```python
from build123d import *

# Parameters (mm, degrees)
F0_W     = 4
F0_H     = 14
F1_DEPTH = 6
F2_R     = 0.8
F3_W     = 7.9375
F3_H     = 6
F4_DEPTH = 6
F5_W     = 7.9375
F5_H     = 6
F6_DEPTH = 6
F8_DEPTH = 25.4


with BuildPart() as f1:
    # F0 (on Front) → F1 (new body)
    with BuildSketch(Plane.XZ):
        Polygon((50.8, 38.1), (-50.8, 38.1), (-50.8, 0), (-20.35, 0), (-20.35, 19.7), (20.35, 19.7), (20.35, 0), (50.8, 0), align=None)
        with Locations((-24.5, 9.85)):
            Rectangle(F0_W, F0_H, mode=Mode.SUBTRACT)
        with Locations((24.5, 9.85)):
            Rectangle(F0_W, F0_H, mode=Mode.SUBTRACT)
    extrude(amount=F1_DEPTH)

    # F2
    f2_edges = [f1.edges().sort_by_distance(p)[0] for p in [
        (-26.5, -3, 16.85),
        (-22.5, -3, 2.85),
        (-22.5, -3, 16.85),
        (-26.5, -3, 2.85),
        (22.5, -3, 2.85),
        (22.5, -3, 16.85),
        (26.5, -3, 16.85),
        (26.5, -3, 2.85),
    ]]
    fillet(f2_edges, radius=F2_R)

    # F3 (on face) → F4 (join)
    with BuildSketch(Plane(origin=(0, 0, 0), x_dir=(1, 0, 0), z_dir=(0, 0, -1))):
        with Locations((-46.83125, 3)):
            Rectangle(F3_W, F3_H)
        with Locations((46.83125, 3)):
            Rectangle(F3_W, F3_H)
        with Locations((-26.19375, 3)):
            Rectangle(F3_W, F3_H)
        with Locations((26.19375, 3)):
            Rectangle(F3_W, F3_H)
    extrude(amount=F4_DEPTH)

    # F5 (on face) → F6 (join)
    with BuildSketch(Plane.XY.offset(38.1)):
        with Locations((-46.83125, -3)):
            Rectangle(F5_W, F5_H)
        with Locations((-26.19375, -3)):
            Rectangle(F5_W, F5_H)
        with Locations((26.19375, -3)):
            Rectangle(F5_W, F5_H)
        with Locations((46.83125, -3)):
            Rectangle(F5_W, F5_H)
    extrude(amount=F6_DEPTH)

    # F7 (on face) → F8 (cut)
    with BuildSketch(Plane.XZ.offset(6)):
        Polygon((-33.2625, 38.1), (-36.5125, 38.1), (-39.7625, 38.1), (-39.7625, 32.1), (-42.8625, 32.1), (-42.8625, 27.1), (-39.7625, 27.1), (-39.7625, 25.1), (-36.5125, 25.1), (-33.2625, 25.1), (-33.2625, 27.1), (-30.1625, 27.1), (-30.1625, 32.1), (-33.2625, 32.1), align=None)
        Polygon((39.7625, 32.1), (39.7625, 38.1), (36.5125, 38.1), (33.2625, 38.1), (33.2625, 32.1), (30.1625, 32.1), (30.1625, 27.1), (33.2625, 27.1), (33.2625, 25.1), (36.5125, 25.1), (39.7625, 25.1), (39.7625, 27.1), (42.8625, 27.1), (42.8625, 32.1), align=None)
        Polygon((33.2625, 6), (33.2625, 0), (36.5125, 0), (39.7625, 0), (39.7625, 6), (42.8625, 6), (42.8625, 11), (39.7625, 11), (39.7625, 13), (36.5125, 13), (33.2625, 13), (33.2625, 11), (30.1625, 11), (30.1625, 6), align=None)
        Polygon((-39.7625, 6), (-39.7625, 0), (-36.5125, 0), (-33.2625, 0), (-33.2625, 6), (-30.1625, 6), (-30.1625, 11), (-33.2625, 11), (-33.2625, 13), (-36.5125, 13), (-39.7625, 13), (-39.7625, 11), (-42.8625, 11), (-42.8625, 6), align=None)
    extrude(amount=-F8_DEPTH, mode=Mode.SUBTRACT)


solid = f1.part
```
Work out the finished part from the listing and answer in its coordinate system (mm). A direction names the side the tool comes from. Give positions to 0.01 mm unless a question says otherwise; leave off trailing zeros. Write each loop counter-clockwise with the first axis right and the second up, starting at its lowest first coordinate (ties: lowest second). Pieces come first, ordered by that corner, then holes.
(1) The part is cut by section A-A on z = -1.5. Write down the section's boundary in (x, y) (1 decimal), plus the area to 4 significant figures.
Final values:
outline: (-50.8, -6) - (-42.9, -6) - (-42.9, 0) - (-50.8, 0) - close; (-30.2, -6) - (-22.2, -6) - (-22.2, 0) - (-30.2, 0) - close; (22.2, -6) - (30.2, -6) - (30.2, 0) - (22.2, 0) - close; (42.9, -6) - (50.8, -6) - (50.8, 0) - (42.9, 0) - close
area: 190.5 mm2
(2) Flat-ended cylindrical pins translate along their axes: pin 1 Ø8 at (x, z) = (-29.5, 17.5) entering from +Y; pin 2 Ø1.5 at (x, y) = (41, -3) entering from +Z; pin 3 Ø1.6 at (x, y) = (-31.5, -2) entering from -Z. Find the tip coordinate at first contact, or state that the pin passes through.
Final values:
pin 1: stops at y = 0
pin 2: stops at z = 38.1
pin 3: stops at z = 0
(3) The mould has two halves that part along Z. Classify faces 1 (the flat face through (-33.262, -3, 3)), 2 (the flat face through (0, -3, 19.7)), 3 (the flat face through (-41, -3, 11)): pulls with the +Z half, pulls with the -Z half, needs draft (parallel to the pull), parting line crosses it, or undercut.
Final values:
face 1: needs draft
face 2: pulls with the -Z half
face 3: undercut
(4) The part is cut by section B-B on y = -4.2. Count the separate pieces of the cut face and the enclosed holes in it, plus the area to 3 significant figures.
Final values:
separate pieces: 1
enclosed holes: 2
area: 2,880 mm2
(5) Which of the six approach directions +Z, -Z, +X, -X, +Y, -Y give full straight-line access (tool end or side, diameter ignored) to faces 4 (the flat face through (20.35, -3, 10)), 5 (the flat face through (42.862, -3, 30)), 6 (the flat face through (-33.262, -3, 35)), 7 (the flat face through (50.8, -3, 19))?
Final values:
face 4: -Z, +Y, -Y
face 5: +Y, -Y
face 6: +Z, +Y, -Y
face 7: +Z, -Z, +X, +Y, -Y
(6) The part is cut by section C-C on x = -7. Write down the section's boundary in (y, z).
Final values:
outline: (-6, 19.7) - (0, 19.7) - (0, 38.1) - (-6, 38.1) - close
(7) Straight lines are drawn through the part: line 1 (X direction, y = -3.6, z = 10); line 2 (X direction, y = -4.7, z = 2); line 3 (X direction, y = -4.3, z = -4) (1 decimal). For each, find the intervals that lie inside material, in ascending order.
Final values:
line 1: x = -50.8 to -42.86, -30.16 to -26.5, -22.5 to -20.35, 20.35 to 22.5, 26.5 to 30.16, 42.86 to 50.8
line 2: x = -50.8 to -39.76, -33.26 to -20.35, 20.35 to 33.26, 39.76 to 50.8
line 3: x = -50.8 to -42.9, -30.2 to -22.2, 22.2 to 30.2, 42.9 to 50.8
